Can you work these out from the model? Positions are in its coordinate system, mm. Give positions to 0.01 mm unless a question says otherwise; leave off trailing zeros. Order: outer loops, then holes, each group sorted by start corner. A loop starts at its lowest first (then second) coordinate and runs counter-clockwise, first axis right, second up. Notation, with made-up numbers: (-28.75, 67) - (19.25, 67) arc R21 cw to (19.25, 100) - close; hole circle Ø11 at (79.25, 53). An arc over 180 degrees is marked (long way). Use one line per item in the form item = value. Start each with the question number.
1) Suppose I cut it at A-A, the plane y = -89. Write out the boundary of the cut face in (x, z), and give its area (3 significant figures).
2) For pin 1 (3 mm diameter, centred on x = 4.5, y = -77, fed in from +Z); pin 2 (2 mm diameter, centred on x = -5.5, z = -4.5, fed in from -Y); pin 3 (1.5 mm diameter, centred on y = -73.5, z = -6, fed in from -X), each with a flat end and sliding along its axis, tell me the tip position at first contact or that it passes through.
3) Suppose I cut it at B-B, the plane x = -8.25. Write out the boundary of the cut face in (y, z), and give its area (3 significant figures).
4) Suppose I cut it at C-C, the plane z = 0. Write out the boundary of the cut face in (x, y).
5) Please list where these lines run through material, in increasing order: probe 1 along X at (y, z) = (-149, 0.75); probe 2 along Z at (x, y) = (2.75, -68); probe 3 along X at (y, z) = (-164, 2.5).
```python
from build123d import *

# Parameters (mm, degrees)
F1_R      = 12.7
F2_DEPTH  = 225.933
F6_W      = 114.097729
F6_H      = 88.5094
F7_DEPTH  = 25.4
F11_W     = 145.65833
F11_H     = 82.475946
F12_DEPTH = 25.4


with BuildPart() as f2:
    # F1 (on face) → F2 (new body)
    with BuildSketch(Plane.XZ):
        Circle(F1_R)
    extrude(amount=F2_DEPTH)

    # F6 (on face) → F7 (cut)
    with BuildSketch(Plane(origin=(78.019506, -188.35575, 0), x_dir=(-0.92388, -0.382683, 0), z_dir=(-0.382683, 0.92388, 0))):
        with Locations((118.185877, 2.949333)):
            Rectangle(F6_W, F6_H)
    extrude(amount=-F7_DEPTH, mode=Mode.SUBTRACT)

    # F11 (on face) → F12 (cut)
    with BuildSketch(Plane(origin=(-1.859872, -4.490128, 0), x_dir=(-0.92388, 0.382683, 0), z_dir=(0.382683, 0.92388, 0))):
        Rectangle(F11_W, F11_H)
    extrude(amount=F12_DEPTH, mode=Mode.SUBTRACT)


solid = f2.part
```
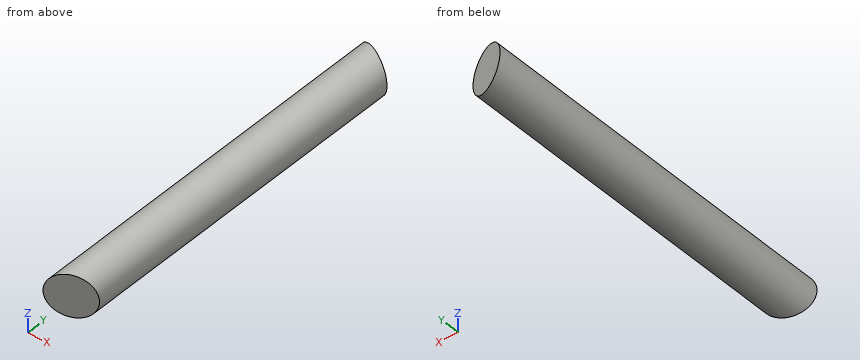
Result sheet:
q1.outline = circle Ø25.4 at (0, 0)
q1.area = 507 mm²
q2.pin_1 = 12.34
q2.pin_2 = -223.36
q2.pin_3 = -11.56
q3.outline = (-224.09, -9.66) - (-1.84, -9.66) - (-1.84, 9.66) - (-224.09, 9.66) - close
q3.area = 4,290 mm²
q4.outline = (-12.7, -225.93) - (12.7, -215.41) - (12.7, -10.52) - (-12.7, 0) - close
q5.probe_1 = -12.68 to 12.68
q5.probe_2 = -12.4 to 12.4
q5.probe_3 = -12.45 to 12.45
